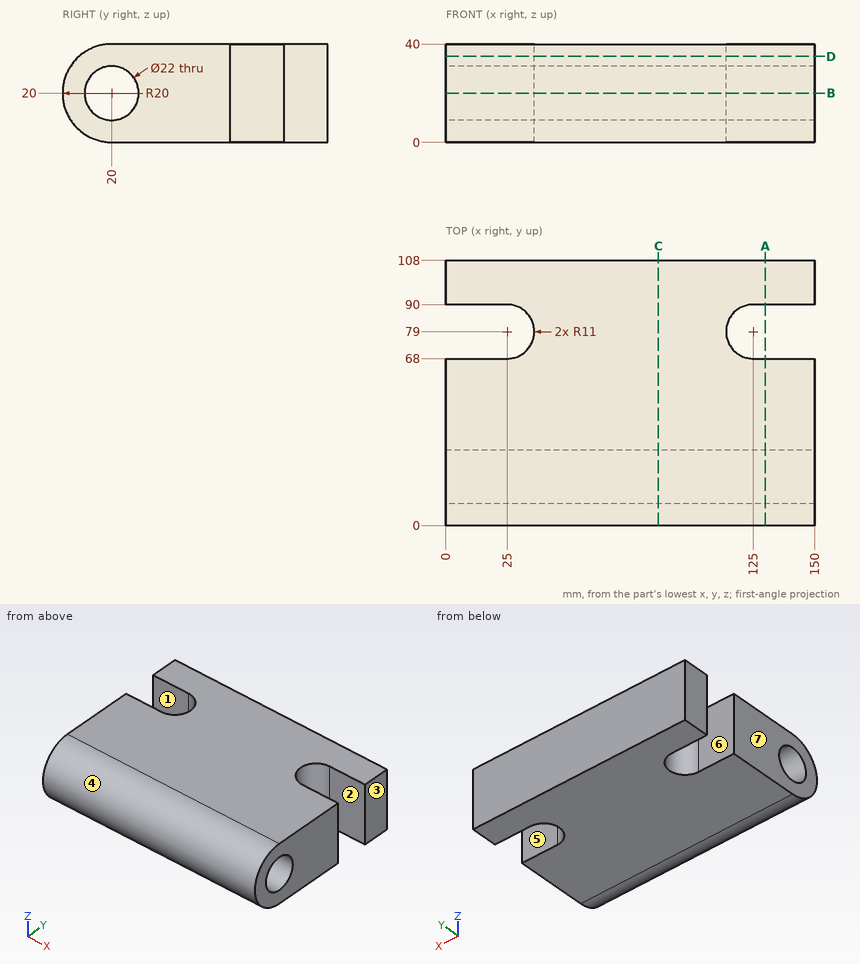
Verification items for this drawing (mm, ordinates from the low corner). A direction names the side the tool comes from. Coordinates: 2 decimals unless noted, no trailing zeros. Order: outer loops, then holes, each group sorted by start corner. A loop starts at its lowest first (then second) coordinate and runs counter-clockwise, first axis right, second up. Notation, with made-up numbers: (34.25, 17) -> (88.25, 17) arc R19 cw to (88.25, 50) -> close; hole circle Ø1 at (10.25, 28.25). An arc over 180 degrees is marked (long way). Put each result on its own line as item: value. Start each with the question number.
1. Cross-section at D-D, the plane z = 35. Record the boundary of the cut face in (x, y), then the cut area to 3 significant figures.
2. Mould release check, pull along Y, two halves, no side actions. Record for the marked faces 4, 5, 6 and 7: released by +Y, released by -Y, zero draft, split by the parting line, or undercut.
3. Material ranges on L1, parallel to Z at x = 44.5, y = 20; L2, parallel to Y at x = 116.5, z = 24; L3, parallel to Y at x = 116, z = 16.5, recorded low to high. Write a range as [from, to].
4. Go/stop test with flat-tipped pins: pin 1 Ø1.5 at (x, y) = (103.5, 12) entering from -Z; pin 2 Ø5 at (x, z) = (35, 33) entering from -Y; pin 3 Ø1 at (x, z) = (111, 20.5) entering from -Y. Record where each tip stops, or that it passes through.
5. Cross-section at C-C, the plane x = 86.5. Record the boundary of the cut face in (y, z), then the cut area to 3 significant figures.
6. Access from +Z, -Z, +X, -X, +Y, -Y to the whole of each face (thin tool, end or side, straight path). Record for the marked faces 1, 2 and 3.
7. Cross-section at B-B, the plane z = 20. Record the boundary of the cut face in (x, y).
8. Cross-section at A-A, the plane x = 130. Record the boundary of the cut face in (y, z), then the cut area to 3 significant figures.
Computed:
1. outline: (0, 6.77) -> (150, 6.77) -> (150, 68) -> (125, 68) arc R11 cw to (125, 90) -> (150, 90) -> (150, 108) -> (0, 108) -> (0, 90) -> (25, 90) arc R11 cw to (25, 68) -> (0, 68) -> close
1. area: 13,700 mm2
2. face 4: released by -Y
2. face 5: undercut
2. face 6: undercut
2. face 7: zero draft
3. L1: [0, 9], [31, 40]
3. L2: [0.4, 9.75], [30.25, 72.02], [85.98, 108]
3. L3: [0.31, 9.57], [30.43, 72.68], [85.32, 108]
4. pin 1: z = 1.36
4. pin 2: y = 2.98
4. pin 3: y = 0
5. outline: (20, 0) -> (108, 0) -> (108, 40) -> (20, 40) arc R20 ccw to start; hole circle Ø22 at (20, 20)
5. area: 3,770 mm2
6. face 1: +Z, -Z, -X
6. face 2: +Z, -Z, +X
6. face 3: +Z, -Z, +X, +Y, -Y
7. outline: (0, 0) -> (150, 0) -> (150, 9) -> (0, 9) -> close; (0, 31) -> (150, 31) -> (150, 68) -> (125, 68) arc R11 cw to (125, 90) -> (150, 90) -> (150, 108) -> (0, 108) -> (0, 90) -> (25, 90) arc R11 cw to (25, 68) -> (0, 68) -> close
8. outline: (20, 0) -> (68, 0) -> (68, 40) -> (20, 40) arc R20 ccw to start; (90, 0) -> (108, 0) -> (108, 40) -> (90, 40) -> close; hole circle Ø22 at (20, 20)
8. area: 2,890 mm2
